```python
from build123d import *

# Parameters (mm, degrees)
SKETCH1_R           = 3.1
SKETCH1_R_2         = 1.65
BOSS_EXTRUDE1_DEPTH = 4.5
BOSS_EXTRUDE2_DEPTH = 15
BOSS_EXTRUDE3_DEPTH = 14
CUT_EXTRUDE1_DEPTH  = 11
SKETCH5_R           = 1.65
CUT_EXTRUDE2_DEPTH  = 73.405110317
CUT_EXTRUDE3_START  = -3
CUT_EXTRUDE3_DEPTH  = 8
FILLET1_R           = 5
SKETCH7_R           = 2.1
CUT_EXTRUDE4_DEPTH  = 47.44243749
SKETCH8_R           = 4.1
CUT_EXTRUDE5_DEPTH  = 1.5
CHAMFER1_SIZE       = 2
CUT_EXTRUDE6_DEPTH  = 64.154572281
CUT_EXTRUDE7_DEPTH  = 64.154572281
SKETCH11_R          = 1.65
CUT_EXTRUDE9_DEPTH  = 64.154572281
BOSS_EXTRUDE4_START = 2
SKETCH13_R          = 2.75
SKETCH13_R_2        = 1.65
BOSS_EXTRUDE4_DEPTH = 2
BOSS_EXTRUDE5_START = 0.825
BOSS_EXTRUDE5_DEPTH = 0.825
CHAMFER3_SIZE       = 2
SKETCH14_R          = 6.1
CUT_EXTRUDE10_DEPTH = 0.7
CHAMFER4_SIZE       = 3
CHAMFER5_SIZE       = 0.83
SKETCH16_R          = 3.4
CUT_EXTRUDE11_DEPTH = 0.5
CHAMFER6_SIZE       = 1.8
CUT_EXTRUDE12_DEPTH = 55.171025466
SKETCH18_R          = 6.25
CUT_EXTRUDE13_DEPTH = 3
FILLET2_R           = 1


# Some blends are built 0.0001 mm under size
with BuildPart() as part:
    # Sketch1 → Boss-Extrude1 (new body)
    with BuildSketch(Plane.XY):
        with BuildLine():
            Line((-10, 17), (-10, -17))
            ThreePointArc((-10, -17), (-9.121320344, -19.121320344), (-7, -20))
            Line((-7, -20), (57.7, -20))
            Line((57.7, -20), (57.7, 20))
            Line((57.7, 20), (10, 20))
            Line((10, 20), (-7, 20))
            ThreePointArc((-7, 20), (-9.121320344, 19.121320344), (-10, 17))
        make_face()
        with Locations((0, 10)):
            Circle(SKETCH1_R, mode=Mode.SUBTRACT)
        with Locations((0, -10)):
            Circle(SKETCH1_R, mode=Mode.SUBTRACT)
        with Locations((30, 8)):
            Circle(SKETCH1_R_2, mode=Mode.SUBTRACT)
    extrude(amount=BOSS_EXTRUDE1_DEPTH)

    # Sketch2 → Boss-Extrude2 (add)
    with BuildSketch(Plane.XZ.offset(20)):
        Polygon((10, 0), (10, -16), (19, -16), (57.7, 0), align=None)
    extrude(amount=-BOSS_EXTRUDE2_DEPTH)

    # Sketch3 → Boss-Extrude3 (add)
    with BuildSketch(Plane(origin=(57.7, 0, 0), x_dir=(0, 0, -1), z_dir=(1, 0, 0))):
        with BuildLine():
            Line((-9.1, 6), (-4.5, 6))
            Line((-4.5, 6), (-4.5, -20))
            Line((-4.5, -20), (-14.862521583, -4.974084173))
            ThreePointArc((-14.862521583, -4.974084173), (-15.297523264, 2.254336399), (-9.1, 6))
        make_face()
    extrude(amount=-BOSS_EXTRUDE3_DEPTH)

    # Sketch4 → Cut-Extrude1 (cut)
    with BuildSketch(Plane(origin=(0, -5, 0), x_dir=(1, 0, 0), z_dir=(0, 1, 0))):
        Polygon((10, 0), (57.7, 0), (57.7, 16), (19, 16), (19, 5.1), (10, 5.1), align=None)
    extrude(amount=-CUT_EXTRUDE1_DEPTH, mode=Mode.SUBTRACT)

    # Sketch5 → Cut-Extrude2 (cut, through all)
    with BuildSketch(Plane(origin=(57.7, 0, 0), x_dir=(0, 0, -1), z_dir=(1, 0, 0))):
        with Locations(Location((-9.1, -1, 0), (0, 0, 90))):
            Circle(SKETCH5_R)
    extrude(amount=-CUT_EXTRUDE2_DEPTH, mode=Mode.SUBTRACT)

    # Sketch6 → Cut-Extrude3 (cut)
    with BuildSketch(Plane(origin=(57.7, 0, 0), x_dir=(0, 0, -1), z_dir=(1, 0, 0)).offset(CUT_EXTRUDE3_START)):
        with BuildLine():
            Line((-5.210912703, -4.889087297), (-19.214201662, -18.892376255))
            Line((-19.214201662, -18.892376255), (-19.214201662, 16.892376255))
            Line((-19.214201662, 16.892376255), (-5.210912703, 2.889087297))
            ThreePointArc((-5.210912703, 2.889087297), (-3.6, -1), (-5.210912703, -4.889087297))
        make_face()
    extrude(amount=-CUT_EXTRUDE3_DEPTH, mode=Mode.SUBTRACT)

    # Fillet1
    fillet1_edges = [part.edges().sort_by_distance(p)[0] for p in [
        (14.5, -5, -16),
    ]]
    fillet(fillet1_edges, radius=FILLET1_R)

    # Sketch7 → Cut-Extrude4 (cut, through all)
    with BuildSketch(Plane(origin=(19, 0, 0), x_dir=(0, 0, -1), z_dir=(1, 0, 0))):
        with Locations(Location((11, -10, 0), (0, 0, 90))):
            Circle(SKETCH7_R)
    extrude(amount=-CUT_EXTRUDE4_DEPTH, mode=Mode.SUBTRACT)

    # Sketch8 → Cut-Extrude5 (cut)
    with BuildSketch(Plane(origin=(19, 0, 0), x_dir=(0, 0, -1), z_dir=(1, 0, 0))):
        with Locations(Location((11, -10, 0), (0, 0, 90))):
            Circle(SKETCH8_R)
    extrude(amount=-CUT_EXTRUDE5_DEPTH, mode=Mode.SUBTRACT)

    # Chamfer1
    chamfer1_edges = [part.edges().sort_by_distance(p)[0] for p in [
        (17.5, -12.1, -11),
    ]]
    chamfer(chamfer1_edges, length=CHAMFER1_SIZE - 0.0001)  # a hair under: the kernel refuses the full size

    # Sketch9 → Cut-Extrude6 (cut, through all)
    with BuildSketch(Plane.XY):
        Polygon((46.7, 6), (54.7, 6), (54.7, 3.5), (54.7, -5.5), (54.7, -8), (46.7, -8), (46.7, -5.5), (46.7, 3.5), align=None)
    extrude(amount=CUT_EXTRUDE6_DEPTH, mode=Mode.SUBTRACT)

    # Sketch10 → Cut-Extrude7 (cut, through all)
    with BuildSketch(Plane(origin=(0, 0, 0), x_dir=(-1, 0, 0), z_dir=(0, 0, -1))):
        with BuildLine():
            Line((-57.7, 6), (-57.7, 20))
            Line((-57.7, 20), (-30, 20))
            ThreePointArc((-30, 20), (-31.436169615, 19.913749067), (-32.851694068, 19.65623614))
            Line((-32.851694068, 19.65623614), (-50.33995445, 15.377739394))
            ThreePointArc((-50.33995445, 15.377739394), (-55.640268278, 11.96054248), (-57.7, 6))
        make_face()
    extrude(amount=-CUT_EXTRUDE7_DEPTH, mode=Mode.SUBTRACT)

    # Sketch11 → Cut-Extrude9 (cut, through all)
    with BuildSketch(Plane(origin=(0, 0, 0), x_dir=(-1, 0, 0), z_dir=(0, 0, -1))):
        with Locations((-16, 15)):
            Circle(SKETCH11_R)
        with Locations((-28, -10)):
            Circle(SKETCH11_R)
    extrude(amount=-CUT_EXTRUDE9_DEPTH, mode=Mode.SUBTRACT)

    # Sketch13 → Boss-Extrude4 (add)
    with BuildSketch(Plane(origin=(46.7, 0, 0), x_dir=(0, 0, -1), z_dir=(1, 0, 0)).offset(BOSS_EXTRUDE4_START)):
        with Locations(Location((-9.1, -1, 0), (0, 0, 90))):
            Circle(SKETCH13_R)
        with Locations(Location((-9.1, -1, 0), (0, 0, 90))):
            Circle(SKETCH13_R_2, mode=Mode.SUBTRACT)
    boss_extrude4 = extrude(amount=-BOSS_EXTRUDE4_DEPTH)

    # Sketch15 → Boss-Extrude5 (add)
    with BuildSketch(Plane(origin=(46.7, 0, 0), x_dir=(0, 0, -1), z_dir=(1, 0, 0)).offset(BOSS_EXTRUDE5_START)):
        with BuildLine():
            Line((-14.078955714, 0.5), (-15.937397166, 0.5))
            ThreePointArc((-15.937397166, 0.5), (-16.1, -1), (-15.937397166, -2.5))
            Line((-15.937397166, -2.5), (-14.078955714, -2.5))
            ThreePointArc((-14.078955714, -2.5), (-14.3, -1), (-14.078955714, 0.5))
        make_face()
    boss_extrude5 = extrude(amount=-BOSS_EXTRUDE5_DEPTH)

    # Mirror1: Boss-Extrude4, Boss-Extrude5 across plane
    add(boss_extrude4.mirror(Plane(origin=(50.7, 0, 0), x_dir=(0, 0, 1), z_dir=(1, 0, 0))))
    add(boss_extrude5.mirror(Plane(origin=(50.7, 0, 0), x_dir=(0, 0, 1), z_dir=(1, 0, 0))))

    # Chamfer3
    chamfer3_edges = [part.edges().sort_by_distance(p)[0] for p in [
        (46.7, -3.75, 9.1),
        (54.7, -3.75, 9.1),
    ]]
    chamfer(chamfer3_edges, length=CHAMFER3_SIZE - 0.0001)  # a hair under: the kernel refuses the full size

    # Sketch14 → Cut-Extrude10 (cut)
    with BuildSketch(Plane(origin=(0, 0, 4.5), x_dir=(-1, 0, 0), z_dir=(0, 0, -1))):
        with Locations((0, -10)):
            Circle(SKETCH14_R)
        with Locations((0, 10)):
            Circle(SKETCH14_R)
    extrude(amount=CUT_EXTRUDE10_DEPTH, mode=Mode.SUBTRACT)

    # Chamfer4
    chamfer4_edges = [part.edges().sort_by_distance(p)[0] for p in [
        (-3.1, -10, 3.8),
        (-3.1, 10, 3.8),
    ]]
    chamfer(chamfer4_edges, length=CHAMFER4_SIZE - 0.0001)  # a hair under: the kernel refuses the full size

    # Chamfer5
    # the kernel refuses this chamfer: 0.83 mm, written as the material it takes off along each edge
    with BuildSketch(Plane(origin=(53.875, -2.5, 18.071894046), x_dir=(0.9996219169112968, -0.027495876610586414, 0), z_dir=(0, 0, -1))) as chamfer5_piece_1_section:
        Polygon((CHAMFER5_SIZE * 0.999621916911, -CHAMFER5_SIZE * 0.0274958766106), (-CHAMFER5_SIZE * 0.0274958766106, -CHAMFER5_SIZE * 0.999621916911), (0, 0), align=None)
    chamfer5_piece_1 = extrude(amount=6.127435212, mode=Mode.PRIVATE)
    chamfer5_piece_1 = split(chamfer5_piece_1, bisect_by=Plane(origin=(54.7, -2.224603208, 15.069483683), z_dir=(-1, 0, 0)), keep=Keep.TOP, mode=Mode.PRIVATE)
    chamfer5_piece_1 = chamfer5_piece_1 - Plane(origin=(54.15228648, -1, 9.1), x_dir=(0, -0.2884615384615384, 0.957491483423431), z_dir=(-1, 0, 0)) * Cylinder(5.2, 16, mode=Mode.PRIVATE)
    add(chamfer5_piece_1, mode=Mode.SUBTRACT)
    with BuildSketch(Plane(origin=(53.875, 0.5, 11.944458834), x_dir=(0.9996219169112968, 0.027495876610586546, 0), z_dir=(0, 0, 1))) as chamfer5_piece_2_section:
        Polygon((CHAMFER5_SIZE * 0.999621916911, -CHAMFER5_SIZE * 0.0274958766106), (-CHAMFER5_SIZE * 0.0274958766106, -CHAMFER5_SIZE * 0.999621916911), (0, 0), align=None)
    chamfer5_piece_2 = extrude(amount=6.127435212, mode=Mode.PRIVATE)
    chamfer5_piece_2 = split(chamfer5_piece_2, bisect_by=Plane(origin=(54.7, 0.224603208, 15.069483683), z_dir=(-1, 0, 0)), keep=Keep.TOP, mode=Mode.PRIVATE)
    chamfer5_piece_2 = chamfer5_piece_2 - Plane(origin=(54.15228648, -1, 9.1), x_dir=(0, -0.2884615384615384, 0.957491483423431), z_dir=(-1, 0, 0)) * Cylinder(5.2, 16, mode=Mode.PRIVATE)
    add(chamfer5_piece_2, mode=Mode.SUBTRACT)
    with BuildSketch(Plane(origin=(47.525, -2.5, 18.071894046), x_dir=(-0.9996219169112968, -0.027495876610586414, 0), z_dir=(0, 0, -1))) as chamfer5_piece_3_section:
        Polygon((CHAMFER5_SIZE * 0.999621916911, CHAMFER5_SIZE * 0.0274958766106), (-CHAMFER5_SIZE * 0.0274958766106, CHAMFER5_SIZE * 0.999621916911), (0, 0), align=None)
    chamfer5_piece_3 = extrude(amount=6.127435212, mode=Mode.PRIVATE)
    chamfer5_piece_3 = split(chamfer5_piece_3, bisect_by=Plane(origin=(46.7, -2.224603208, 15.069483683), z_dir=(1, 0, 0)), keep=Keep.TOP, mode=Mode.PRIVATE)
    chamfer5_piece_3 = chamfer5_piece_3 - Plane(origin=(47.24771352, -1, 9.1), x_dir=(0, -0.2884615384615384, 0.957491483423431), z_dir=(1, 0, 0)) * Cylinder(5.2, 16, mode=Mode.PRIVATE)
    add(chamfer5_piece_3, mode=Mode.SUBTRACT)
    with BuildSketch(Plane(origin=(47.525, 0.5, 11.944458834), x_dir=(-0.9996219169112968, 0.027495876610586285, 0), z_dir=(0, 0, 1))) as chamfer5_piece_4_section:
        Polygon((CHAMFER5_SIZE * 0.999621916911, CHAMFER5_SIZE * 0.0274958766106), (-CHAMFER5_SIZE * 0.0274958766106, CHAMFER5_SIZE * 0.999621916911), (0, 0), align=None)
    chamfer5_piece_4 = extrude(amount=6.127435212, mode=Mode.PRIVATE)
    chamfer5_piece_4 = split(chamfer5_piece_4, bisect_by=Plane(origin=(46.7, 0.224603208, 15.069483683), z_dir=(1, 0, 0)), keep=Keep.TOP, mode=Mode.PRIVATE)
    chamfer5_piece_4 = chamfer5_piece_4 - Plane(origin=(47.24771352, -1, 9.1), x_dir=(0, -0.2884615384615384, 0.957491483423431), z_dir=(1, 0, 0)) * Cylinder(5.2, 16, mode=Mode.PRIVATE)
    add(chamfer5_piece_4, mode=Mode.SUBTRACT)

    # Sketch16 → Cut-Extrude11 (cut)
    with BuildSketch(Plane(origin=(0, 0, 4.5), x_dir=(-1, 0, 0), z_dir=(0, 0, -1))):
        with Locations((-28, -10)):
            Circle(SKETCH16_R)
        with Locations((-16, 15)):
            Circle(SKETCH16_R)
    extrude(amount=CUT_EXTRUDE11_DEPTH, mode=Mode.SUBTRACT)

    # Chamfer6
    # the kernel refuses this chamfer: 1.8 mm, written as the material it takes off along each edge
    with BuildSketch(Plane(origin=(28, -10, 4), x_dir=(-1, 0, 0), z_dir=(0, -1, 0))) as chamfer6_piece_1_section:
        Polygon((1.65, CHAMFER6_SIZE), (1.65 + CHAMFER6_SIZE, 0), (1.65, 0), align=None)
    chamfer6_piece_1 = revolve(axis=Axis((28, -10, 4), (0, 0, -1)), mode=Mode.PRIVATE)
    chamfer6_piece_1 = chamfer6_piece_1 & Plane(origin=(28, -10, 3.070206715), x_dir=(-1, 0, 0), z_dir=(0, 0, 1)) * Cylinder(3.4, 14, mode=Mode.PRIVATE)
    add(chamfer6_piece_1, mode=Mode.SUBTRACT)
    with BuildSketch(Plane(origin=(16, 15, 4), x_dir=(-1, 0, 0), z_dir=(0, -1, 0))) as chamfer6_piece_2_section:
        Polygon((1.65, CHAMFER6_SIZE), (1.65 + CHAMFER6_SIZE, 0), (1.65, 0), align=None)
    chamfer6_piece_2 = revolve(axis=Axis((16, 15, 4), (0, 0, -1)), mode=Mode.PRIVATE)
    chamfer6_piece_2 = chamfer6_piece_2 & Plane(origin=(16, 15, 3.070206715), x_dir=(-1, 0, 0), z_dir=(0, 0, 1)) * Cylinder(3.4, 14, mode=Mode.PRIVATE)
    add(chamfer6_piece_2, mode=Mode.SUBTRACT)

    # Sketch17 → Cut-Extrude12 (cut, through all)
    with BuildSketch(Plane.ZY.offset(-10)):
        Polygon((-11, -10), (-9.51507576, -8.51507576), (-10.550151519, -7.48), (-11.449848481, -7.48), (-12.48492424, -8.51507576), align=None)
    extrude(amount=-CUT_EXTRUDE12_DEPTH, mode=Mode.SUBTRACT)

    # Sketch18 → Cut-Extrude13 (cut)
    with BuildSketch(Plane(origin=(0, 0, 0), x_dir=(-1, 0, 0), z_dir=(0, 0, -1))):
        with Locations((-30, 8)):
            Circle(SKETCH18_R)
    extrude(amount=-CUT_EXTRUDE13_DEPTH, mode=Mode.SUBTRACT)

    # Fillet2
    fillet2_edges = [part.edges().sort_by_distance(p)[0] for p in [
        (46.7, 6, 2.25),
        (54.7, 6, 2.25),
    ]]
    fillet(fillet2_edges, radius=FILLET2_R)


solid = part.part
```
Input: part model. Units: mm. Frame: model coordinates. A direction names the side the tool comes from. Coordinates: 2 decimals unless noted, no trailing zeros. Loops run counter-clockwise (first coordinate to the right, second up) from the corner with the lowest first, then second, coordinate; pieces in that order, holes last. Notation, with made-up numbers: (66.25, -1) - (83.25, -1) arc R15 cw to (83.25, 8) - close; hole circle Ø2 at (9, -3.5). An arc over 180 degrees is marked (long way). Answer in a Markdown table with one row per item.
(1) Cut plane C-C on z = -2. Output: boundary loops of the cut face in (x, y).
Model answer:
| item | result |
|---|---|
| outline | (10, -20) - (52.86, -20) - (52.86, -16) - (10, -16) - close |
(2) Cut plane D-D on x = 41. Output: boundary loops of the cut face in (y, z), plus the area to 3 significant figures.
Model answer:
| item | result |
|---|---|
| outline | (-20, -6.9) - (-16, -6.9) - (-16, 0) - (17.66, 0) - (17.66, 4.5) - (-20, 4.5) - close |
| area | 197 mm² |
(3) Cut plane A-A on x = 8. Output: boundary loops of the cut face in (y, z).
Model answer:
| item | result |
|---|---|
| outline | (-20, 0) - (20, 0) - (20, 4.5) - (-20, 4.5) - close |
(4) Cut plane B-B on y = 8. Count the separate pieces of the cut face and the enclosed holes in it, plus the area to 3 significant figures.
Model answer:
| item | result |
|---|---|
| separate pieces | 3 |
| enclosed holes | 0 |
| area | 225 mm² |
(5) Material intervals for L1, parallel to Z at x = 14, y = -10; L2, parallel to Y at x = 30, z = 1.6; L3, parallel to Y at x = 0, z = 0.55, sorted ascending. Write a range as from..to.
Model answer:
| item | result |
|---|---|
| L1 | z = -16..-13.1, -8.9..-5.1, 0..4.5 |
| L2 | y = -20..1.75, 14.25..20 |
| L3 | y = -20..-13.1, -6.9..6.9, 13.1..20 |
(6) Mould query, pull axis Z, two halves, no side actions, for faces 1 (the face through (16, 0, 4.5)), 2 (the face through (55.2, -1.4, 7.5)), 3 (the face through (53.875, -1, 15)). Classes: pulls with the +Z half, pulls with the -Z half, needs draft (parallel to the pull), parting line crosses it, or undercut.
Model answer:
| item | result |
|---|---|
| face 1 | pulls with the +Z half |
| face 2 | undercut |
| face 3 | needs draft |
(7) Set-up query: faces 4 (the face through (52.825, 1.742, 9.964)), 5 (the face through (51, -8, 4)), 6 (the face through (31.355, 1.899, 1.479)). Return all of +Z, -Z, +X, -X, +Y, -Y with unobstructed straight access to the full face (end or side cutting, diameter ignored); none if empty.
Model answer:
| item | result |
|---|---|
| face 4 | none |
| face 5 | +Z, -Z |
| face 6 | -Z |
(8) Pin query (flat end, axial travel): P1, Ø9, axis at x = 16, y = 15, coming from the -Z side; P2, Ø8, axis at x = 38, y = 3.5, coming from the +Z side; P3, Ø4.5, axis at y = -1, z = 10.5, coming from the -X side. Return the tip coordinate at first contact, or that it passes through.
Model answer:
| item | result |
|---|---|
| P1 | stops at z = 0 |
| P2 | stops at z = 4.5 |
| P3 | stops at x = 43.7 |
